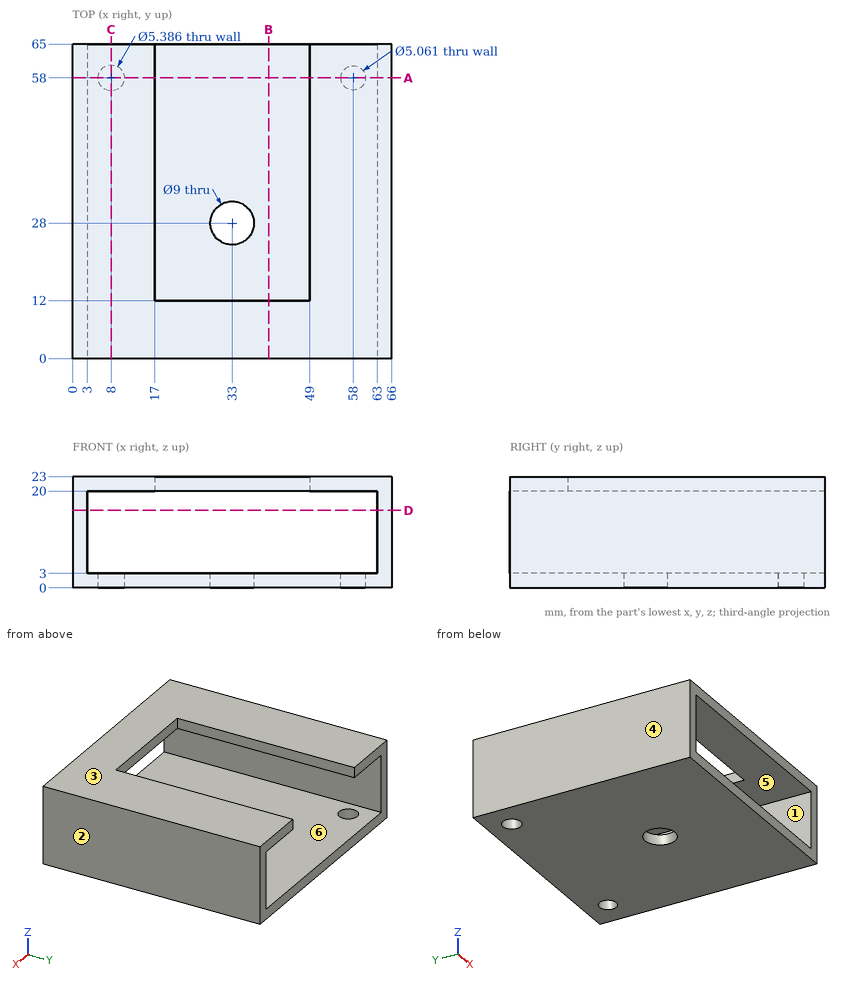
Can you work these out from the drawing? Everything is in mm from the part's minimum corner. A direction names the side the tool comes from. Give positions to 0.01 mm unless a question says otherwise; leave off trailing zeros. Order: outer loops, then holes, each group sorted by start corner. A loop starts at its lowest first (then second) coordinate and runs counter-clockwise, first axis right, second up. Notation, with made-up numbers: M -21,-15 L 14,-15 A15 cw 14,-5 Z; hole C 2.5,28 d5. An arc over 180 degrees is marked long. Write item = value, one per line. Start each with the question number.
Q1. I need wall thicknesses on probe 1 along X at (y, z) = (19, 21.5); probe 2 along Z at (x, y) = (51.5, 60); probe 3 along Y at (x, z) = (33, 1.45). Which ranges of each line are inside material? Lowest first, please. Write a range as [from, to].
Q2. For the marked faces 1 and 2, which set-ups out of +Z, -Z, +X, -X, +Y, -Y let a thin tool reach every point of the face, with its end or its side?
Q3. Will these pins go through, and if not, where does the flat tip stop? pin 1 Ø6 at (y, z) = (10, 20.5) entering from -X; pin 2 Ø1 at (x, y) = (42, 37) entering from +Z; pin 3 Ø2.5 at (x, z) = (26, 21.5) entering from +Y.
Q4. Suppose I cut it at C-C (x = 8). Write out the boundary of the cut face in (y, z), plus the area to 3 significant figures.
Q5. Suppose I cut it at A-A (y = 58). Write out the boundary of the cut face in (x, z).
Q6. Suppose I cut it at B-B (x = 40.5). Write out the boundary of the cut face in (y, z).
Q7. Suppose I cut it at D-D (z = 16). Write out the boundary of the cut face in (x, y), plus the area to 3 significant figures.
Q8. We'd pull the mould along X, two halves only. Please class the marked faces 3, 4, 5 and 6: pulls with the +X half, pulls with the -X half, needs draft (parallel to the pull), parting line crosses it, or undercut.
Check result:
q1.probe_1 = [0, 17], [49, 66]
q1.probe_2 = [0, 3], [20, 23]
q1.probe_3 = [0, 23.5], [32.5, 65]
q2.face_1 = +Y, -Y
q2.face_2 = +Z, -Z, +X, +Y, -Y
q3.pin_1 = 0
q3.pin_2 = 3
q3.pin_3 = 12
q4.outline = M 0,0 L 55.31,0 L 55.31,3 L 0,3 Z; M 0,20 L 65,20 L 65,23 L 0,23 Z; M 60.69,0 L 65,0 L 65,3 L 60.69,3 Z
q4.area = 374 mm2
q5.outline = M 0,0 L 5.31,0 L 5.31,3 L 3,3 L 3,20 L 17,20 L 17,23 L 0,23 Z; M 10.69,0 L 55.47,0 L 55.47,3 L 10.69,3 Z; M 49,20 L 63,20 L 63,3 L 60.53,3 L 60.53,0 L 66,0 L 66,23 L 49,23 Z
q6.outline = M 0,0 L 65,0 L 65,3 L 0,3 Z; M 0,20 L 12,20 L 12,23 L 0,23 Z
q7.outline = M 0,0 L 3,0 L 3,65 L 0,65 Z; M 63,0 L 66,0 L 66,65 L 63,65 Z
q7.area = 390 mm2
q8.face_3 = needs draft
q8.face_4 = pulls with the -X half
q8.face_5 = undercut
q8.face_6 = undercut
